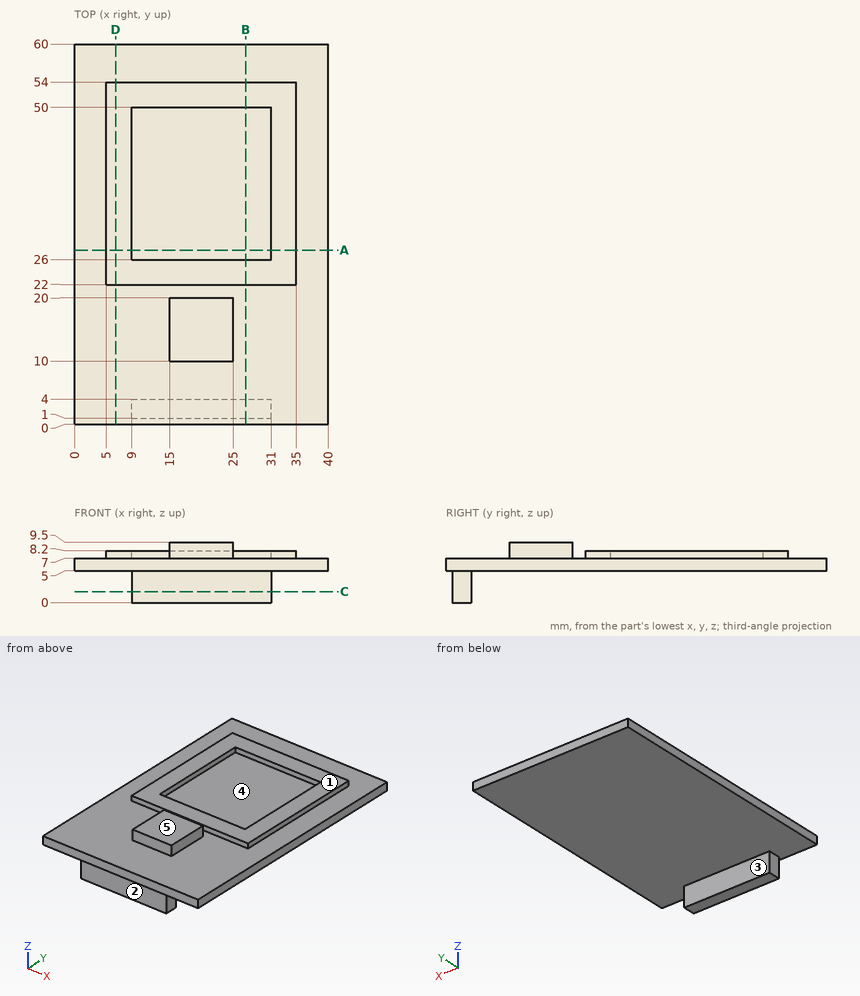
Print and shaded views of the part. All mm, measured from the part's lowest x, y and z. A direction names the side the tool comes from. Coordinates: 2 decimals unless noted, no trailing zeros. Write each loop counter-clockwise with the first axis right and the second up, starting at its lowest first coordinate (ties: lowest second). Pieces come first, ordered by that corner, then holes. Notation, with made-up numbers: M -0.75,-26 L 44.25,-26 A7 ccw 44.25,-13 Z; hole C -23.75,3 d10. An arc over 180 degrees is marked long. Return JSON: item names as keys, results as strings.
1. Saw through at B-B, the plane x = 27. Write the cut outline in (y, z).
Determined:
{"outline": "M 0,5 L 1,5 L 1,0 L 4,0 L 4,5 L 60,5 L 60,7 L 54,7 L 54,8.2 L 50,8.2 L 50,7 L 26,7 L 26,8.2 L 22,8.2 L 22,7 L 0,7 Z"}
2. Saw through at A-A, the plane y = 27.5. Write the cut outline in (x, z).
Determined:
{"outline": "M 0,5 L 40,5 L 40,7 L 35,7 L 35,8.2 L 31,8.2 L 31,7 L 9,7 L 9,8.2 L 5,8.2 L 5,7 L 0,7 Z"}
3. 3-axis set-ups, long thin cutter, end or side, ignore diameter. For the marked faces 1 and 2: which of +Z, -Z, +X, -X, +Y, -Y reach the whole face in a straight line?
Determined:
{"face 1": "+Z, +X, -X, +Y", "face 2": "-Z, +X, -X, -Y"}
4. Flat gauge pins, fed straight in: pin 1 Ø2 at (y, z) = (13.5, 9) entering from -X; pin 2 Ø5 at (y, z) = (17.5, 1.5) entering from +X; pin 3 Ø5.5 at (x, z) = (17.5, 2) entering from -Y; pin 4 Ø0.6 at (x, z) = (23.5, 8) entering from +Y. Where does each tip first touch, or does it go through?
Determined:
{"pin 1": "x = 15", "pin 2": "through", "pin 3": "y = 1", "pin 4": "y = 54"}
5. Saw through at D-D, the plane x = 6.5. Write the cut outline in (y, z), then the cut area to 3 significant figures.
Determined:
{"outline": "M 0,5 L 60,5 L 60,7 L 54,7 L 54,8.2 L 22,8.2 L 22,7 L 0,7 Z", "area": "158 mm²"}
6. Probe L1, parallel to Y at x = 28.5, z = 8; L2, parallel to Z at x = 20.5, y = 21; L3, parallel to Y at x = 28, z = 2.75. List the from-to ranges inside material, lowest first.
Determined:
{"L1": "22 to 26, 50 to 54", "L2": "5 to 7", "L3": "1 to 4"}
7. Pull direction Y, two halves, no side cores. Call the marked faces 3, 4 and 5: pulls with the +Y half, pulls with the -Y half, needs draft (parallel to the pull), parting line crosses it, or undercut.
Determined:
{"face 3": "pulls with the +Y half", "face 4": "undercut", "face 5": "needs draft"}
8. Saw through at C-C, the plane z = 1.75. Write the cut outline in (x, y), then the cut area to 3 significant figures.
Determined:
{"outline": "M 9,1 L 31,1 L 31,4 L 9,4 Z", "area": "66.0 mm²"}
